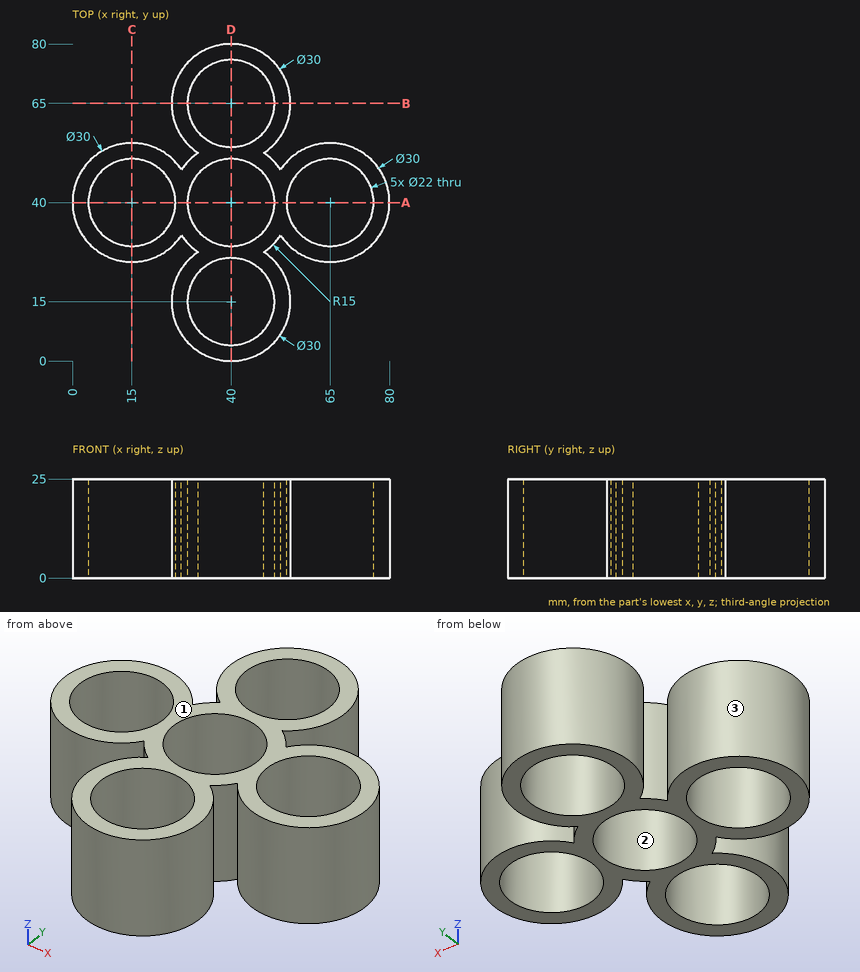
Geometry check sheet. Reference: drawing and pictorial views, mm from the part's lowest x, y, z. Coordinates: 2 decimals unless noted, no trailing zeros. Order: outer loops, then holes, each group sorted by start corner. A loop starts at its lowest first (then second) coordinate and runs counter-clockwise, first axis right, second up. Notation, with made-up numbers: M 12,41.25 L 61,41.25 A33 cw 61,70.25 Z; hole C 64,37 d7. An arc over 180 degrees is marked long. Write each question's results on one line, items separated by ' | '. Start each with the question number.
1. Cross-section at A-A on y = 40. Record the cut outline in (x, z).
2. Material ranges on probe 1 along Y at (x, z) = (39.5, 7.5); probe 2 along Y at (x, z) = (65, 17); probe 3 along X at (y, z) = (45, 21), recorded low to high.
3. Mould release check, pull along X, two halves, no side actions. Record for the marked faces 1, 2 and 3: +X half, -X half, draft (parallel to the pull), parting line (faces both ways), or undercut.
4. Go/stop test with flat-tipped pins: P1, Ø2, axis at x = 69, y = 56.5, coming from the +Z side; P2, Ø1.5, axis at y = 12, z = 10, coming from the -X side; P3, Ø8, axis at x = 34.5, z = 17.5, coming from the +Y side; P4, Ø8, axis at x = 46.5, z = 21, coming from the -Y side. Record where each tip stops, or that it passes through.
5. Cross-section at B-B on y = 65. Record the cut outline in (x, z).
Checks:
1) outline: M 0,0 L 4,0 L 4,25 L 0,25 Z; M 26,0 L 29,0 L 29,25 L 26,25 Z; M 51,0 L 54,0 L 54,25 L 51,25 Z; M 76,0 L 80,0 L 80,25 L 76,25 Z
2) probe 1: y = 0.01 to 4.01, 25.99 to 29.01, 50.99 to 54.01, 75.99 to 79.99 | probe 2: y = 25 to 29, 51 to 55 | probe 3: x = 0.86 to 5.2, 24.8 to 30.2, 49.8 to 55.2, 74.8 to 79.14
3) face 1: draft | face 2: undercut | face 3: undercut
4) P1: passes through | P2: stops at x = 25.17 | P3: stops at y = 79.92 | P4: stops at y = 0.21
5) outline: M 25,0 L 29,0 L 29,25 L 25,25 Z; M 51,0 L 55,0 L 55,25 L 51,25 Z
